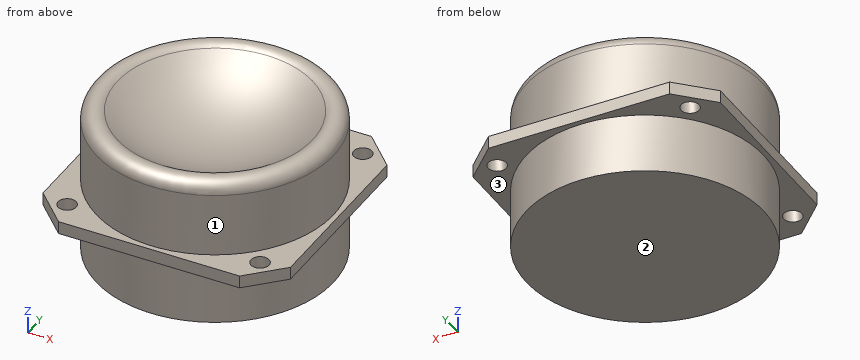
from build123d import *

# Parameters (mm, degrees)
SKETCH1_W                  = 49
SKETCH1_H                  = 49
BOSS_EXTRUDE1_DEPTH        = 2.5
CUT_EXTRUDE1_DEPTH         = 2.5
F_3_6_3_6_DIAMETER_HOLE1_D = 3.6


with BuildPart() as part:
    # Sketch1 → Boss-Extrude1 (new body)
    with BuildSketch(Plane.XY):
        Rectangle(SKETCH1_W, SKETCH1_H)
    extrude(amount=-BOSS_EXTRUDE1_DEPTH)

    # Sketch2 → Revolve1 (revolve)
    with BuildSketch(Plane(origin=(0, 0, 0), x_dir=(0, 0, -1), z_dir=(1, 0, 0))):
        with BuildLine():
            Line((14.29, 0), (14.29, 23.5))
            Line((14.29, 23.5), (-12.55, 23.5))
            ThreePointArc((-12.55, 23.5), (-14.850205099, 22.037337692), (-14.501257994, 19.333902758))
            ThreePointArc((-14.501257994, 19.333902758), (-9.305131525, 10.281048048), (-7.501257994, 0))
            Line((-7.501257994, 0), (14.29, 0))
        make_face()
    revolve(axis=Axis((0, 0, 0), (0, 0, 1)))

    # Sketch3 → Cut-Extrude1 (cut)
    with BuildSketch(Plane.XY):
        Polygon((-24.5, 17.926406871), (-17.926406871, 24.5), (-24.5, 24.5), align=None)
        Polygon((24.5, 17.926406871), (17.926406871, 24.5), (24.5, 24.5), align=None)
        Polygon((-24.5, -17.926406871), (-24.5, -24.5), (-17.926406871, -24.5), align=None)
        Polygon((24.5, -17.926406871), (17.926406871, -24.5), (24.5, -24.5), align=None)
    extrude(amount=-CUT_EXTRUDE1_DEPTH, mode=Mode.SUBTRACT)

    # Ø3.6 (3.6) Diameter Hole1 (through all)
    with Locations(Plane.XY):
        with Locations((-19.091883092, 19.091883092), (19.091883092, -19.091883092), (-19.091883092, -19.091883092), (19.091883092, 19.091883092)):
            Hole(F_3_6_3_6_DIAMETER_HOLE1_D / 2)


solid = part.part
Can you work these out from the model? Positions are in its coordinate system, mm. Face numbers are marked on the shaded views. A direction names the side the tool comes from. Round coordinates to 2 decimals unless told otherwise and drop trailing zeros. Loops run counter-clockwise (first coordinate to the right, second up) from the corner with the lowest first, then second, coordinate; pieces in that order, holes last. Notation, with made-up numbers: (78, 23) - (131, 23) arc R17 ccw to (131, 32) - close; hole circle Ø10 at (83.25, -34). An arc over 180 degrees is marked (long way). Answer in a Markdown table with one row per item. Add a question column.
Q1. I want a section at A-A on y = 0. List the corners of the cut face in (x, z) for me, and give its area (3 significant figures).
Q2. For pin 1 Ø4 at (x, y) = (-19.09, 19.09) entering from -Z; pin 2 Ø2 at (x, z) = (-18, 6.5) entering from +Y (3 decimals); pin 3 Ø5 at (y, z) = (-5.5, 11) entering from +X; pin 4 Ø6 at (y, z) = (-19, -2.5) entering from -X, each with a flat end and sliding along its axis, tell me the tip position at first contact or that it passes through.
Q3. Which directions (+Z, -Z, +X, -X, +Y, -Y) give clear straight access to the entire face, cutting with the end or side of a thin tool? Please do the marked faces 1, 2 and 3.
Q4. I need wall thicknesses on L1, parallel to Z at x = 18.5, y = 22.5; L2, parallel to Z at x = -13, y = 1.5; L3, parallel to Y at x = -9.5, z = -5.25. Which ranges of each line are inside material? Lowest first, please.
Q5. I want a section at C-C on z = -12.5. List the corners of the cut face in (x, y) for me.
A:
| question | item | result |
|---|---|---|
| 1 | outline | (-24.5, -2.5) - (-23.5, -2.5) - (-23.5, -14.29) - (23.5, -14.29) - (23.5, -2.5) - (24.5, -2.5) - (24.5, 0) - (23.5, 0) - (23.5, 12.55) arc R2.54 ccw to (19.33, 14.5) arc R30.2 cw to (-19.33, 14.5) arc R2.54 ccw to (-23.5, 12.55) - (-23.5, 0) - (-24.5, 0) - close |
| 1 | area | 1,170 mm^2 |
| 2 | pin 1 | z = -2.5 |
| 2 | pin 2 | y = 16.225 |
| 2 | pin 3 | x = 23.31 |
| 2 | pin 4 | x = -24.5 |
| 3 | face 1 | +Z |
| 3 | face 2 | -Z, +X, -X, +Y, -Y |
| 3 | face 3 | -Z |
| 4 | L1 | -2.5 to 0 |
| 4 | L2 | -14.29 to 10.48 |
| 4 | L3 | -21.49 to 21.49 |
| 5 | outline | circle Ø47 at (0, 0) |
